Read the model definition and answer for the solid it produces. Units are mm, in the model's axes. Face numbers are marked on the shaded views. A direction names the side the tool comes from. Round coordinates to 2 decimals unless told otherwise and drop trailing zeros. Loops run counter-clockwise (first coordinate to the right, second up) from the corner with the lowest first, then second, coordinate; pieces in that order, holes last. Notation, with made-up numbers: M -18.5,55.5 L -9.5,55.5 A22 ccw -9.5,68.5 Z; hole C 25.5,29 d7. An arc over 180 degrees is marked long. Answer as CSV lines item,"result".
```python
from build123d import *

# Parameters (mm, degrees)
SKETCH_1_R          = 8.5
SKETCH_2_R          = 11
SKETCH_4_R          = 11
CUT_EXTRUDE_1_DEPTH = 36.89599575
SKETCH_10_R         = 7
SKETCH_9_R          = 7
CUT_EXTRUDE_START   = -4.15
SKETCH_12_R         = 7.3
CUT_EXTRUDE_4_DEPTH = 4.15


with BuildPart() as part:
    # Эскиз1 → Loft 1 section 0
    with BuildSketch(Plane(origin=(0, 0, 0), x_dir=(1, 0, 0), z_dir=(0, 1, 0))):
        Circle(SKETCH_1_R)
    # Эскиз2 → Loft 1 section 1
    with BuildSketch(Plane(origin=(0, -4.15, 0), x_dir=(1, 0, 0), z_dir=(0, 1, 0))):
        Circle(SKETCH_2_R)
    loft()

    # Эскиз4 → section 1 of loft_2
    with BuildSketch(Plane(origin=(0, -28.65, 0), x_dir=(1, 0, 0), z_dir=(0, 1, 0)), mode=Mode.PRIVATE) as loft_2_s1:
        Circle(SKETCH_4_R)
    # loft up to a face of the part (loft_2)
    loft([Face(Wire([part.edges().sort_by_distance((-7.530018165, -4.15, 8.018654902))[0]])), loft_2_s1.sketch])

    # Эскиз5 → По сечениям3 section 0
    with BuildSketch(Plane(origin=(0, -28.65, 0), x_dir=(1, 0, 0), z_dir=(0, 1, 0))):
        with BuildLine():
            Line((0, 10), (-8.660254038, 5))
            Line((-8.660254038, 5), (-8.660254038, -5))
            Line((-8.660254038, -5), (0, -10))
            Line((0, -10), (8.660254038, -5))
            Line((8.660254038, -5), (8.660254038, 5))
            Line((8.660254038, 5), (0, 10))
        make_face()
    # Эскиз7 → По сечениям3 section 1
    with BuildSketch(Plane(origin=(0, -32.35, 0), x_dir=(1, 0, 0), z_dir=(0, 1, 0))):
        with BuildLine():
            Line((0, 10), (-8.660254038, 5))
            Line((-8.660254038, 5), (-8.660254038, -5))
            Line((-8.660254038, -5), (0, -10))
            Line((0, -10), (8.660254038, -5))
            Line((8.660254038, -5), (8.660254038, 5))
            Line((8.660254038, 5), (0, 10))
        make_face()
    loft()

    # Эскиз8 → Вырез-Вытянуть1 (cut, through all)
    with BuildSketch(Plane.XZ.offset(32.35)):
        Polygon((-6.062177826, 3.5), (-6.062177826, -3.5), (0, -7), (6.062177826, -3.5), (6.062177826, 3.5), (0, 7), align=None)
    extrude(amount=-CUT_EXTRUDE_1_DEPTH, mode=Mode.SUBTRACT)

    # Эскиз10 → Loft 1 2 section 0
    with BuildSketch(Plane(origin=(0, -12, 0), x_dir=(1, 0, 0), z_dir=(0, 1, 0))):
        Circle(SKETCH_10_R)
    # Эскиз9 → Loft 1 2 section 1
    with BuildSketch(Plane(origin=(0, -20.35, 0), x_dir=(1, 0, 0), z_dir=(0, 1, 0))):
        Circle(SKETCH_9_R)
    loft(mode=Mode.SUBTRACT)

    # Эскиз12 → Вырез-Вытянуть4 (cut)
    with BuildSketch(Plane(origin=(0, 0, 0), x_dir=(1, 0, 0), z_dir=(0, 1, 0)).offset(CUT_EXTRUDE_START)):
        with Locations(Location((0, 0, 0), (0, 0, 270))):
            Circle(SKETCH_12_R)
    extrude(amount=CUT_EXTRUDE_4_DEPTH, mode=Mode.SUBTRACT)


solid = part.part
```
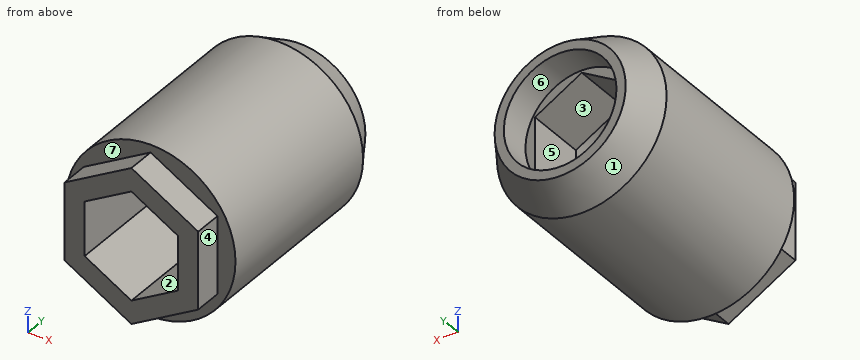
1) Determine the mould class of the marked faces 1, 2, 3 and 4 for opening direction Z: released by +Z, released by -Z, zero draft, split by the parting line, or undercut.
Evaluation:
face 1,"split by the parting line"
face 2,"undercut"
face 3,"undercut"
face 4,"zero draft"
2) A tool of negligible diameter and unlimited length cuts with its end or side. For the marked faces 5, 6 and 7, from which of +Z, -Z, +X, -X, +Y, -Y can it reach the whole face along a straight path? Write none if from no direction.
Evaluation:
face 5,"+Y, -Y"
face 6,"+Y"
face 7,"-Y"
3) Straight lines are drawn through the part: line 1 (Y direction, x = -5, z = -4.25); line 2 (X direction, y = -15, z = 0). For each, find the intervals that lie inside material, in ascending order.
Evaluation:
line 1,"y = -32.35 to -20.35, -12 to -4.15"
line 2,"x = -11 to -7, 7 to 11"
4) Find section B-B, the plane y = -15. Give the vertices of the cut face in (x, z).
Evaluation:
outline,"C 0,0 d22; hole C 0,0 d14"
5) Each of these flat-tipped pins is pushed along its axis until it touches: P1, Ø0.5, axis at x = 6.5, z = -1.5, coming from the +Y side; P2, Ø1.5, axis at x = 7, y = -8, coming from the +Z side; P3, Ø3, axis at y = -26.5, z = -8.5, coming from the -X side. Where does it stop, or does it pass through?
Evaluation:
P1,"stops at y = -4.15"
P2,"stops at z = 9.05"
P3,"stops at x = -8.49"
6) Find section A-A, the plane y = -24.5. Give the vertices of the cut face in (x, z).
Evaluation:
outline,"C 0,0 d22; hole M -6.06,-3.5 L 0,-7 L 6.06,-3.5 L 6.06,3.5 L 0,7 L -6.06,3.5 Z"
